from build123d import *

# Parameters (mm, degrees)
F0_R     = 7.112
F1_DEPTH = 59.563
F2_R     = 9.5758
F2_R_2   = 7.112
F3_DEPTH = 5.842
F5_DEPTH = 5.08


with BuildPart() as f1:
    # F0 (on Front) → F1 (new body)
    with BuildSketch(Plane.XZ):
        Circle(F0_R)
    extrude(amount=F1_DEPTH)

    # F2 (on face) → F3 (join)
    with BuildSketch(Plane.XZ.offset(59.563)):
        Circle(F2_R)
        Circle(F2_R_2, mode=Mode.SUBTRACT)
        Circle(F2_R_2)
    extrude(amount=F3_DEPTH)

    # F4 (on face) → F5 (cut)
    with BuildSketch(Plane.XZ.offset(65.405)):
        Polygon((8.5051758644, 0.2550774705), (4.0316843628, 7.4932370975), (-4.4734915016, 7.238159627), (-8.5051758644, -0.2550774705), (-4.0316843628, -7.4932370975), (4.4734915016, -7.238159627), align=None)
    extrude(amount=-F5_DEPTH, mode=Mode.SUBTRACT)


solid = f1.part
Verification items for the finished model (mm, model axes). A direction names the side the tool comes from. Give positions to 0.01 mm unless a question says otherwise; leave off trailing zeros. Write each loop counter-clockwise with the first axis right and the second up, starting at its lowest first coordinate (ties: lowest second). Pieces come first, ordered by that corner, then holes.
(1) Access from +Z, -Z, +X, -X, +Y, -Y to the whole of each face (thin tool, end or side, straight path). Record for faces 4 (the face through (-6, -65.405, -5)), 5 (the face through (6.461, -62.901, -3.544)), 6 (the face through (-1.46, -59.563, 7.14)).
(2) Gauge pin test, flat ends, axial feed: pin 1 (1.5 mm diameter, centred on y = -11, z = -0.5, fed in from +X); pin 2 (8 mm diameter, centred on x = -2, y = -18, fed in from +Z); pin 3 (3 mm diameter, centred on x = 4, y = -29, fed in from -Z). Record the tip position at first contact, or that the pin passes through.
(3) Cross-section at B-B (y = -58.5). Enter the section's corners in (x, z).
(4) Material ranges on line 1 (Y direction, x = 6.75, z = -5) (3 decimals); line 2 (Y direction, x = -5.5, z = 3.25) (3 decimals); line 3 (Z direction, x = -0.75, y = -51), recorded low to high.
(5) Mould release check, pull along X, two halves, no side actions. Record for faces 1 (the face through (0, 0, 0)), 2 (the face through (-6.3, -62.9, -3.82)), 3 (the face through (-1.542, -29.365, -6.943)): +X half, -X half, draft (parallel to the pull), parting line (faces both ways), or undercut.
(6) Cross-section at A-A (x = 6.5). Enter the section's corners in (y, z) (3 decimals), plus the area to 3 significant figures.
(7) Cross-section at C-C (z = 1.75). Enter the section's corners in (x, y) (3 decimals).
Worked out:
1. face 4: +Z, -Z, +X, -X, -Y
1. face 5: -Y
1. face 6: +Y
2. pin 1: stops at x = 7.11
2. pin 2: stops at z = 7.11
2. pin 3: stops at z = -6.66
3. outline: circle Ø14.22 at (0, 0)
4. line 1: y = -65.405 to -59.563
4. line 2: y = -60.325 to 0
4. line 3: z = -7.07 to 7.07
5. face 1: draft
5. face 2: undercut
5. face 3: parting line
6. outline: (-65.405, -7.032) - (-59.563, -7.032) - (-59.563, -2.886) - (0, -2.886) - (0, 2.886) - (-59.563, 2.886) - (-59.563, 7.032) - (-65.405, 7.032) - (-65.405, 3.499) - (-60.325, 3.499) - (-60.325, -3.472) - (-65.405, -3.472) - close
6. area: 391 mm2
7. outline: (-9.415, -65.405) - (-7.426, -65.405) - (-7.426, -60.325) - (7.581, -60.325) - (7.581, -65.405) - (9.415, -65.405) - (9.415, -59.563) - (6.893, -59.563) - (6.893, 0) - (-6.893, 0) - (-6.893, -59.563) - (-9.415, -59.563) - close
